from build123d import *

# Parameters (mm, degrees)
CROQUIS1_R                 = 10
CROQUIS1_R_2               = 2.65
SALIENTE_EXTRUIR1_DEPTH    = 30
CROQUIS2_R                 = 1.7
CORTAR_EXTRUIR1_DEPTH      = 30
CROQUIS3_W                 = 6
CROQUIS3_H                 = 3
CORTAR_EXTRUIR2_DEPTH      = 9
CORTAR_EXTRUIR3_DEPTH      = 34.166248054
CORTAR_EXTRUIR3_DEPTH_BACK = 34.166248054


with BuildPart() as part:
    # Croquis1 → Saliente-Extruir1 (new body)
    with BuildSketch(Plane(origin=(0, 0, 0), x_dir=(1, 0, 0), z_dir=(0, 1, 0))):
        with Locations(Location((0, 0, 0), (0, 0, 270))):
            Circle(CROQUIS1_R)
        with Locations(Location((0, 0, 0), (0, 0, 270))):
            Circle(CROQUIS1_R_2, mode=Mode.SUBTRACT)
    extrude(amount=SALIENTE_EXTRUIR1_DEPTH)

    # Croquis2 → Cortar-Extruir1 (cut)
    with BuildSketch(Plane.XY):
        with Locations(Location((0, 5.5, 0), (0, 0, 180))):
            Circle(CROQUIS2_R)
    extrude(amount=CORTAR_EXTRUIR1_DEPTH, mode=Mode.SUBTRACT)

    # Croquis3 → Cortar-Extruir2 (cut)
    with BuildSketch(Plane(origin=(0, 0, 0), x_dir=(-1, 0, 0), z_dir=(0, -1, 0))):
        with Locations((0, -5.5)):
            Rectangle(CROQUIS3_W, CROQUIS3_H)
    extrude(amount=-CORTAR_EXTRUIR2_DEPTH, mode=Mode.SUBTRACT)

    # Croquis4 → Cortar-Extruir3 (cut, two sides: drawn at the far end of the back side and taken through both)
    with BuildSketch(Plane.XY.offset(-CORTAR_EXTRUIR3_DEPTH_BACK)):
        Polygon((0, 17.443375673), (-1.25, 16.721687836), (-1.25, 15.278312164), (0, 14.556624327), (1.25, 15.278312164), (1.25, 16.721687836), align=None)
        Polygon((0, 25.443375673), (-1.25, 24.721687836), (-1.25, 23.278312164), (0, 22.556624327), (1.25, 23.278312164), (1.25, 24.721687836), align=None)
    extrude(amount=CORTAR_EXTRUIR3_DEPTH + CORTAR_EXTRUIR3_DEPTH_BACK, mode=Mode.SUBTRACT)

    # Croquis5 → Cortar-Revolución1 (revolve, cut)
    with BuildSketch(Plane.XY, mode=Mode.PRIVATE) as cortar_revoluci_n1_sk:
        with BuildLine():
            Line((-10, 27), (-10, 21))
            ThreePointArc((-10, 21), (-8.5, 24), (-10, 27))
        make_face()
        with BuildLine():
            Line((-10, 19), (-10, 13))
            ThreePointArc((-10, 13), (-8.5, 16), (-10, 19))
        make_face()
    revolve(cortar_revoluci_n1_sk.sketch.rotate(Axis((0, 16, 0), (0, 1, 0)), 180), axis=Axis((0, 16, 0), (0, 1, 0)), mode=Mode.SUBTRACT)


solid = part.part
The model under review builds one solid part; all positions refer to its coordinate system, in mm. A direction names the side the tool comes from. Round coordinates to 2 decimals unless told otherwise and drop trailing zeros. Order: outer loops, then holes, each group sorted by start corner. A loop starts at its lowest first (then second) coordinate and runs counter-clockwise, first axis right, second up. Notation, with made-up numbers: (85, 50.25) - (119, 50.25) arc R34 ccw to (119, 87.25) - close; hole circle Ø11 at (-35, 49.5). An arc over 180 degrees is marked (long way). Use one line per item in the form item = value.
Q1. To check wall thickness, follow line 1 (Z direction, x = 0, y = 8.5); line 2 (X direction, y = 9, z = 0); line 3 (Y direction, x = 7, z = 6). State the ranges of each line that lie inside material, in increasing order.
Response values:
line_1 = -10 to -2.65, 2.65 to 4, 7 to 10
line_2 = -10 to -2.65, 2.65 to 10
line_3 = 0 to 13.79, 18.21 to 21.79, 26.21 to 30
Q2. Mouldability with a two-part tool opening along Y and no side actions: class faces 1 (the flat face through (0, 9, 5)), 2 (the flat face through (-0.63, 22.92, -5.61)), 3 (the flat face through (0, 3, 4)) as pulls with the +Y half, pulls with the -Y half, needs draft (parallel to the pull), parting line crosses it, or undercut.
Response values:
face_1 = pulls with the -Y half
face_2 = undercut
face_3 = needs draft
Q3. Tool access review of faces 4 (the flat face through (0, 3, 7)), 5 (the flat face through (-0.616, 17.088, 5.518)), 6 (the cylindrical face through (0.37, 7.16, 8.48)): name each direction out of +Z, -Z, +X, -X, +Y, -Y from which nothing blocks a thin tool from reaching the whole face with its end or side.
Response values:
face_4 = -Y
face_5 = +Z, -Z
face_6 = +Z
Q4. Add section A-A on z = 0. Give the boundary of the cut face in (x, y), then the cut area to 3 significant figures.
Response values:
outline = (-10, 0) - (-2.65, 0) - (-2.65, 30) - (-10, 30) - (-10, 27) arc R3.75 cw to (-10, 21) - (-10, 19) arc R3.75 cw to (-10, 13) - close; (2.65, 0) - (10, 0) - (10, 13) arc R3.75 cw to (10, 19) - (10, 21) arc R3.75 cw to (10, 27) - (10, 30) - (2.65, 30) - close
area = 416 mm^2
Q5. Add section D-D on y = 20.5. Give the boundary of the cut face in (x, z), then the cut area to 3 significant figures.
Response values:
outline = circle Ø20 at (0, 0); hole circle Ø5.3 at (0, 0)
area = 292 mm^2
Q6. Clearance check with flat-ended pins moving along their axes: P1, Ø2.5, axis at x = 0, z = 5.5, coming from the -Y side; P2, Ø2.5, axis at y = 4.5, z = 5, coming from the -X side; P3, Ø0.7, axis at y = 24, z = 5, coming from the -X side; P4, Ø5, axis at x = 0, z = 0, coming from the +Y side. State where each tip first meets the part, or that it passes through.
Response values:
P1 = 9
P2 = -9.27
P3 = -7.12
P4 = through
Q7. Add section C-C on y = 16. Give the boundary of the cut face in (x, z).
Response values:
outline = (-1.25, -8.41) - (-1.25, -2.34) arc R2.65 cw to (-1.25, 2.34) - (-1.25, 8.41) arc R8.5 ccw to start; (1.25, -8.41) arc R8.5 ccw to (1.25, 8.41) - (1.25, 2.34) arc R2.65 cw to (1.25, -2.34) - close
Q8. Add section B-B on y = 8.5. Give the boundary of the cut face in (x, z).
Response values:
outline = circle Ø20 at (0, 0); hole (-3, 4) - (3, 4) - (3, 7) - (-3, 7) - close; hole circle Ø5.3 at (0, 0)
